Autodesk Inventor part; units mm, degrees
ref_plane "YZ Plane" through (0, 0, 0) normal (1, 0, 0) x (0, 1, 0)
ref_plane "XZ Plane" through (0, 0, 0) normal (0, 1, 0) x (-1, 0, 0)
ref_plane "XY Plane" through (0, 0, 0) normal (0, 0, 1) x (1, 0, 0)
ref_plane "Work Plane1" through (0, 0, 0) normal (0, 0, -1) x (-1, 0, 0)
sketch "Sketch3" plane through (0, 0, 0) normal (0, 0, -1) x (-1, 0, 0)
  circle A0 centre (0, 0) radius 11
  line L0 (-15.4, 0) -> (15.4, 0)
  dimension "d19" = 22
extrude "Extrusion3" add sketch "Sketch3" against normal blind 3.6
sketch "Sketch4" plane through (0, 0, 3.6) normal (0, 0, 1) x (1, 0, 0)
  arc A0 (10.583, -3) -> (10.583, 3) centre (0, 0) ccw
  line L0 (-16.2075, 0) -> (20.2449, 0)
  line L1 (15, 0) -> (15, 2)
  arc A1 (15, 2) -> (10.583, 3) centre (9.5173, -11.9621) ccw
  line L2 (15, 0) -> (15, -2)
  arc A2 (10.583, -3) -> (15, -2) centre (9.5173, 11.9621) ccw
  dimension "d22" = 2
  dimension "d23" = 3
  dimension "d24" = 15
  dimension "d25" = 15
  dimension "d35" = 11
extrude "Extrusion4" add sketch "Sketch4" against normal blind 3.6
sketch "Sketch2" plane through (0, 0, 0) normal (0, 0, -1) x (-1, 0, 0)
  line L0 (-9.8, -2.6) -> (-6, -2.6)
  line L1 (-6, -2.6) -> (-6, 2.6)
  line L2 (-6, 2.6) -> (-9.8, 2.6)
  line L3 (-9.8, 2.6) -> (-9.8, -2.6)
  line L4 (-9.8, -2.6) -> (-6, 2.6) construction
  line L5 (-6, -2.6) -> (-9.8, 2.6) construction
  line L6 (0, -27.5637) -> (0, 32.5752)
  line L7 (9.8, -2.6) -> (6, -2.6)
  line L8 (6, -2.6) -> (6, 2.6)
  line L9 (6, 2.6) -> (9.8, 2.6)
  line L10 (9.8, 2.6) -> (9.8, -2.6)
  line L11 (9.8, -2.6) -> (6, 2.6) construction
  line L12 (6, -2.6) -> (9.8, 2.6) construction
  circle A0 centre (-7.9, 0) radius 1.625
  circle A1 centre (7.9, 0) radius 1.625
  point P0 (0, 0)
  dimension "d31" = 6
  dimension "d32" = 0
  dimension "d33" = 3.25
  dimension "d34" = 3.25
extrude "Extrusion2" cut sketch "Sketch2" against normal blind 3.6 contours A0 | A1
pattern_circular "Circular Pattern1" count 8 over 360 about axis through (0, 0, 0) along (0, 0, 1) of "Extrusion4"
properties part number "tandwiel(ja)"
For this review, take the finished solid that the model builds, in its own axes (mm). A direction names the side the tool comes from. Coordinates: 2 decimals unless noted, no trailing zeros. Write each loop counter-clockwise with the first axis right and the second up, starting at its lowest first coordinate (ties: lowest second). Pieces come first, ordered by that corner, then holes.
(1) Add section D-D on y = 7. Give the boundary of the cut face in (x, z), then the cut area to 3 significant figures.
(2) Add section B-B on z = 0.4. Count the separate pieces of the cut face and the enclosed holes in it, then the cut area to 3 significant figures.
(3) Tool access review of faces 1 (the face through (4.226, -10.156, 1.775)), 2 (the face through (12.86, 2.66, 1.83)), 3 (the face through (-2.66, 12.86, 1.83)): name each direction out of +Z, -Z, +X, -X, +Y, -Y from which nothing blocks a thin tool from reaching the whole face with its end or side.
(4) For pin 1 Ø3 at (x, y) = (-7.9, 0) entering from +Z; pin 2 Ø1.5 at (x, z) = (8, 1) entering from -Y; pin 3 Ø1.5 at (y, z) = (-5, 3) entering from +X, all flat-tipped, find the tip position at first contact; note any pin that passes through.
(5) Add section A-A on y = 0. Give the boundary of the cut face in (x, z) (3 decimals).
(6) Add section C-C on x = -7.9. Give the boundary of the cut face in (y, z) (3 decimals), then the cut area to 3 significant figures.
(7) Wall thickness on probe 1 along X at (y, z) = (-0.5, 1); probe 2 along X at (y, z) = (1, 0.55); probe 3 along Y at (x, z) = (7.9, 0.8) (3 decimals): over which ranges is each line inside the solid? List them lowest first.
Answer sheet:
1. outline: (-10.84, 0) - (10.84, 0) - (10.84, 3.6) - (-10.84, 3.6) - close
1. area: 78.0 mm2
2. separate pieces: 1
2. enclosed holes: 2
2. area: 535 mm2
3. face 1: +Z, -Z, -Y
3. face 2: +Z, -Z, +X
3. face 3: +Z, -Z, +Y
4. pin 1: passes through
4. pin 2: stops at y = -11.82
4. pin 3: stops at x = 10.15
5. outline: (-15, 0) - (-9.525, 0) - (-9.525, 3.6) - (-15, 3.6) - close; (-6.275, 0) - (6.275, 0) - (6.275, 3.6) - (-6.275, 3.6) - close; (9.525, 0) - (15, 0) - (15, 3.6) - (9.525, 3.6) - close
6. outline: (-11.382, 0) - (-1.625, 0) - (-1.625, 3.6) - (-11.382, 3.6) - close; (1.625, 0) - (11.382, 0) - (11.382, 3.6) - (1.625, 3.6) - close
6. area: 70.2 mm2
7. probe 1: x = -15 to -9.45, -6.35 to 6.35, 9.45 to 15
7. probe 2: x = -15 to -9.18, -6.62 to 6.62, 9.18 to 15
7. probe 3: y = -11.382 to -1.625, 1.625 to 11.382
